Source: CAD feature listing. Evaluate the final solid. Frame: model axes, mm. A direction names the side the tool comes from. Give positions to 0.01 mm unless a question says otherwise; leave off trailing zeros. Order: outer loops, then holes, each group sorted by start corner. A loop starts at its lowest first (then second) coordinate and runs counter-clockwise, first axis right, second up. Notation, with made-up numbers: M 14,0.25 L 47,0.25 A18 cw 47,9.25 Z; hole C 79.5,18 d2. An arc over 180 degrees is marked long. Return JSON: item names as keys, results as strings.
Autodesk Inventor part; units mm, degrees
ref_plane "YZ Plane" through (0, 0, 0) normal (1, 0, 0) x (0, 1, 0)
ref_plane "XZ Plane" through (0, 0, 0) normal (0, 1, 0) x (-1, 0, 0)
ref_plane "XY Plane" through (0, 0, 0) normal (0, 0, 1) x (1, 0, 0)
sketch "Sketch1" plane through (0, 0, 0) normal (0, 1, 0) x (-1, 0, 0)
  circle A0 centre (0, 0) radius 6.35
  dimension "d0" = 12.7
extrude "Extrusion1" add sketch "Sketch1" along normal blind 254
thread "Thread1"
sketch "Sketch2" plane through (0, 254, 0) normal (0, 1, 0) x (1, 0, 0)
  circle A0 centre (0, 0) radius 6.35
  arc A1 (1.7227, -2.667) -> (-1.7227, -2.667) centre (0, 0) ccw
  line L0 (-1.7227, -2.667) -> (1.7227, -2.667)
  dimension "d5" = 6.35
  dimension "d6" = 2.667
extrude "Extrusion2" cut sketch "Sketch2" against normal blind 9.525
sketch "Sketch3" plane through (0, 0, 0) normal (0, -1, 0) x (1, 0, 0)
  circle A0 centre (0, 0) radius 6.35
  circle A1 centre (0, 0) radius 5
  dimension "d9" = 10
extrude "Extrusion3" cut sketch "Sketch3" against normal blind 19.05
properties part number "acmeScrew"
1. Ray query, probe 1 along Y at (x, z) = (-4, -1.25) (3 decimals); probe 2 along Z at (x, y) = (-0.5, 142); probe 3 along Z at (x, y) = (5.5, 158). Return the intervals inside material, ascending.
Evaluation:
{"probe 1": "y = 0 to 244.475", "probe 2": "z = -6.33 to 6.33", "probe 3": "z = -3.17 to 3.17"}
2. Set-up query: faces 1 (the face through (0, 0, 0)), 2 (the face through (0, 244.475, 3)), 3 (the face through (-1.08, 9.39, -4.88)). Return all of +Z, -Z, +X, -X, +Y, -Y with unobstructed straight access to the full face (end or side cutting, diameter ignored); none if empty.
Evaluation:
{"face 1": "+Z, -Z, +X, -X, -Y", "face 2": "+Y", "face 3": "-Y"}
3. Draft query along Y for faces 4 (the face through (0, 254, 0)), 5 (the face through (1.38, 130.18, 6.2)), 6 (the face through (2, 19.05, -5)). Return one class per face: pulls with the +Y half, pulls with the -Y half, needs draft (parallel to the pull), parting line crosses it, or undercut.
Evaluation:
{"face 4": "pulls with the +Y half", "face 5": "needs draft", "face 6": "pulls with the -Y half"}
4. Section query B-B (y = 177). Return loops of the section in (x, z).
Evaluation:
{"outline": "C 0,0 d12.7"}
5. Section query A-A (z = 0). Return loops of the section in (x, y) (3 decimals), then the cut area to 3 significant figures.
Evaluation:
{"outline": "M -6.35,19.05 L -5,19.05 L -5,0 L 5,0 L 5,19.05 L 6.35,19.05 L 6.35,244.475 L 3.175,244.475 L 3.175,254 L -3.175,254 L -3.175,244.475 L -6.35,244.475 Z", "area": "3,110 mm^2"}
6. First-contact query: pin 1 (2 mm diameter, centred on y = 173, z = -2.5, fed in from +X); pin 2 (1 mm diameter, centred on x = -1, y = 102, fed in from +Z); pin 3 (1 mm diameter, centred on y = 148.5, z = -1.5, fed in from -X). Flat tips, straight axial feed; report the tip coordinate or a pass-through.
Evaluation:
{"pin 1": "stops at x = 6.17", "pin 2": "stops at z = 6.33", "pin 3": "stops at x = -6.27"}
